Source: CAD feature listing. Evaluate the final solid. Frame: model axes, mm. Round coordinates to 2 decimals unless told otherwise and drop trailing zeros. Write each loop counter-clockwise with the first axis right and the second up, starting at its lowest first coordinate (ties: lowest second). Pieces come first, ordered by that corner, then holes. Notation, with made-up numbers: M 72,5.5 L 103,5.5 A16 cw 103,19.5 Z; hole C -34,3.25 d7. An arc over 180 degrees is marked long. Use a Markdown table: item, result.
```python
from build123d import *

# Parameters (mm, degrees)
F0_W     = 105
F0_H     = 115
F0_R     = 2.5
F1_DEPTH = 3
F2_SIZE2 = 2.5
F2_SIZE  = 2.5


with BuildPart() as f1:
    # F0 (on Top) → F1 (new body)
    with BuildSketch(Plane.XY):
        with Locations((0, 2)):
            Rectangle(F0_W, F0_H)
        with Locations((-45, -45)):
            Circle(F0_R, mode=Mode.SUBTRACT)
        with Locations((45, -45)):
            Circle(F0_R, mode=Mode.SUBTRACT)
        with Locations((-45, 45)):
            Circle(F0_R, mode=Mode.SUBTRACT)
        with Locations((-25, 55)):
            Circle(F0_R, mode=Mode.SUBTRACT)
        with Locations((25, 55)):
            Circle(F0_R, mode=Mode.SUBTRACT)
        with Locations((45, 45)):
            Circle(F0_R, mode=Mode.SUBTRACT)
    extrude(amount=F1_DEPTH)

    # F2
    f2_edges = [f1.edges().sort_by_distance(p)[0] for p in [
        (-47.5, -45, 0),
        (42.5, -45, 0),
        (42.5, 45, 0),
        (-47.5, 45, 0),
    ]]
    chamfer(f2_edges, length=F2_SIZE, length2=F2_SIZE2)


solid = f1.part
```
Q1. Line query: L1, parallel to Y at x = 45, z = 2.8; L2, parallel to X at y = -42.5, z = 1.6; L3, parallel to X at y = -46.5, z = 1.3. Output: solid intervals per line, ascending.
Results are:
| item | result |
|---|---|
| L1 | -55.5 to -47.5, -42.5 to 42.5, 47.5 to 59.5 |
| L2 | -52.5 to -47.3, -42.7 to 42.7, 47.3 to 52.5 |
| L3 | -52.5 to -48.38, -41.62 to 41.62, 48.38 to 52.5 |
Q2. Section C-C on x = -45. Return loops of the section in (y, z).
Results are:
| item | result |
|---|---|
| outline | M -55.5,0 L -50,0 L -47.5,2.5 L -47.5,3 L -55.5,3 Z; M -42.5,2.5 L -40,0 L 40,0 L 42.5,2.5 L 42.5,3 L -42.5,3 Z; M 47.5,2.5 L 50,0 L 59.5,0 L 59.5,3 L 47.5,3 Z |
Q3. Section A-A on x = -25. Return loops of the section in (y, z), plus the area to 3 significant figures.
Results are:
| item | result |
|---|---|
| outline | M -55.5,0 L 52.5,0 L 52.5,3 L -55.5,3 Z; M 57.5,0 L 59.5,0 L 59.5,3 L 57.5,3 Z |
| area | 330 mm^2 |
Q4. Section B-B on z = 0.8. Return loops of the section in (x, y), plus the area to 3 significant figures.
Results are:
| item | result |
|---|---|
| outline | M -52.5,-55.5 L 52.5,-55.5 L 52.5,59.5 L -52.5,59.5 Z; hole C -45,-45 d8.4; hole C -45,45 d8.4; hole C -25,55 d5; hole C 25,55 d5; hole C 45,-45 d8.4; hole C 45,45 d8.4 |
| area | 11,800 mm^2 |
Q5. First-contact query: pin 1 Ø4.5 at (x, y) = (-45, -45) entering from +Z; pin 2 Ø6 at (x, y) = (45, -45) entering from -Z. Flat tips, straight axial feed; report the tip coordinate or a pass-through.
Results are:
| item | result |
|---|---|
| pin 1 | through |
| pin 2 | z = 2 |
Q6. Mould query, pull axis Y, two halves, no side actions, for faces 1 (the flat face through (-52.5, 1, 1)), 2 (the cylindrical face through (47.31, 44.04, 2.75)), 3 (the flat face through (-1, -55.5, 1)), 4 (the flat face through (-1, 59.5, 1)). Classes: +Y half, -Y half, draft (parallel to the pull), parting line (faces both ways), or undercut.
Results are:
| item | result |
|---|---|
| face 1 | draft |
| face 2 | undercut |
| face 3 | -Y half |
| face 4 | +Y half |
